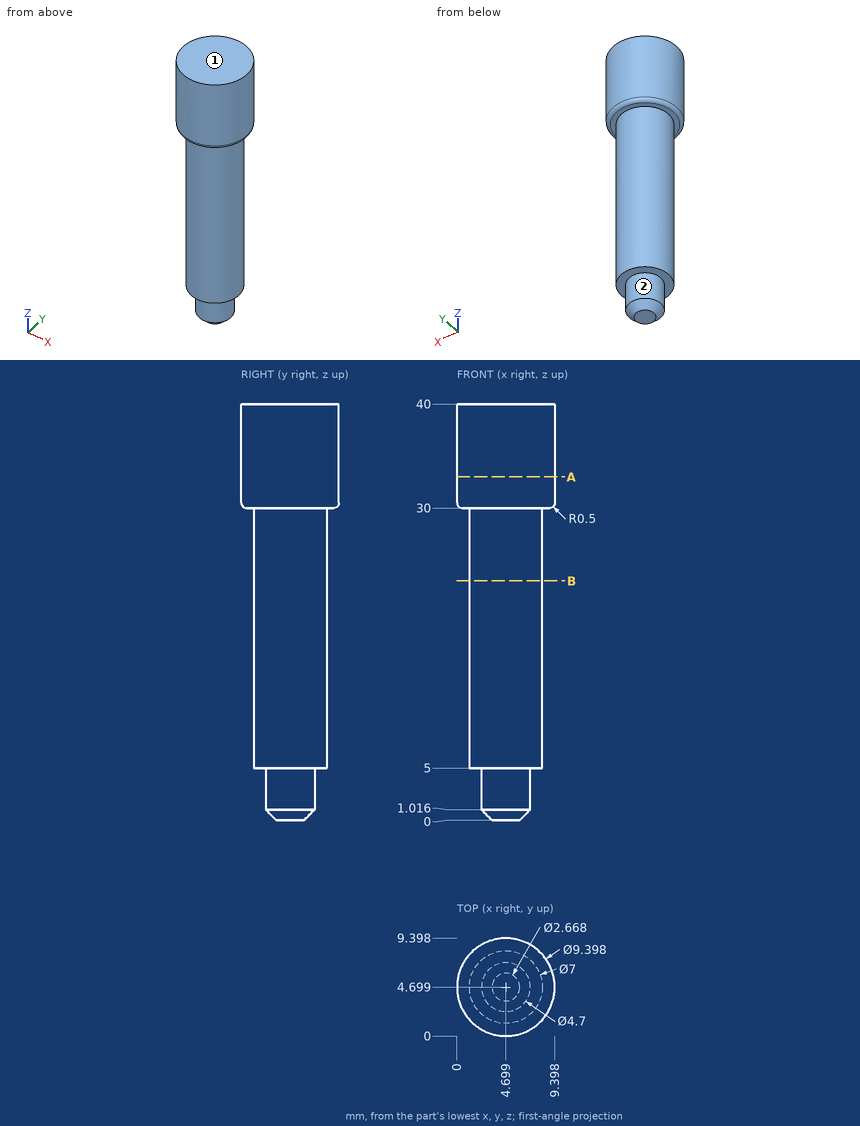
Answer from the drawing. Dimensions are ordinates in mm from the lowest x, y and z of the part. A direction names the side the tool comes from. Give positions to 0.01 mm unless a question says otherwise; leave off trailing zeros. Loops run counter-clockwise (first coordinate to the right, second up) from the corner with the lowest first, then second, coordinate; pieces in that order, holes last. Notation, with made-up numbers: (-1, -2) -> (51, -2) arc R35 cw to (51, 32) -> close; hole circle Ø6 at (86.25, 1.25). An arc over 180 degrees is marked (long way). One line per question, with ' | ' between items. Start each with the question number.
1) Straight lines are drawn through the part: L1, parallel to Z at x = 2.5, y = 6; L2, parallel to Z at x = 2, y = 7; L3, parallel to X at y = 4.5, z = 16.5. For each, find the intervals that lie inside material, in ascending order.
2) Section A-A, the plane z = 33 is taken. Determine the outline of the cut face in (x, y), then the cut area to 3 significant figures.
3) Each of these flat-tipped pins is pushed along its axis until it touches: pin 1 (2 mm diameter, centred on x = 2, z = 15, fed in from -Y); pin 2 (1.5 mm diameter, centred on x = 2, z = 12, fed in from +Y); pin 3 (2 mm diameter, centred on x = 4, z = 9, fed in from -Y). Where does it stop, or does it pass through?
4) Section B-B, the plane z = 23 is taken. Determine the outline of the cut face in (x, y), then the cut area to 3 significant figures.
5) For the marked faces 1 and 2, determine the directions among +Z, -Z, +X, -X, +Y, -Y from which every point of the face is accessible in a straight line to the end or side of a thin tool.
Resolved:
1) L1: 5 to 40 | L2: 30 to 40 | L3: 1.2 to 8.19
2) outline: circle Ø9.4 at (4.7, 4.7) | area: 69.4 mm2
3) pin 1: y = 1.64 | pin 2: y = 7.61 | pin 3: y = 1.2
4) outline: circle Ø7 at (4.7, 4.7) | area: 38.5 mm2
5) face 1: +Z, +X, -X, +Y, -Y | face 2: -Z
